from build123d import *

# Parameters (mm, degrees)
F0_R     = 0.6
F1_DEPTH = 1.7
F3_DEPTH = 2
F5_DEPTH = 1
F6_R     = 1.1
F7_DEPTH = 2.701
F8_R     = 2.35
F9_DEPTH = 2


with BuildPart() as f1:
    # F0 (on Top) → F1 (new body)
    with BuildSketch(Plane.XY):
        with BuildLine():
            ThreePointArc((2.2299103121, -2.5), (3.057180036, -1.369726333), (3.35, 0))
            ThreePointArc((3.35, 0), (3.057180036, 1.369726333), (2.2299103121, 2.5))
            ThreePointArc((2.2299103121, 2.5), (-3.35, 0), (2.2299103121, -2.5))
        make_face()
        with BuildLine():
            ThreePointArc((2.2299103121, 2.5), (3.057180036, 1.369726333), (3.35, 0))
            ThreePointArc((3.35, 0), (3.057180036, -1.369726333), (2.2299103121, -2.5))
            Line((2.2299103121, -2.5), (14, -2))
            ThreePointArc((14, -2), (16, 0), (14, 2))
            Line((14, 2), (2.2299103121, 2.5))
        make_face()
        with Locations((4, 0)):
            Circle(F0_R, mode=Mode.SUBTRACT)
        with Locations((6, 0)):
            Circle(F0_R, mode=Mode.SUBTRACT)
        with Locations((8, 0)):
            Circle(F0_R, mode=Mode.SUBTRACT)
        with Locations((10, 0)):
            Circle(F0_R, mode=Mode.SUBTRACT)
        with Locations((12, 0)):
            Circle(F0_R, mode=Mode.SUBTRACT)
        with Locations((14, 0)):
            Circle(F0_R, mode=Mode.SUBTRACT)
    extrude(amount=F1_DEPTH)

    # F2 (on face) → F3 (join)
    with BuildSketch(Plane.XY.offset(1.7)):
        with BuildLine():
            ThreePointArc((2.2299103121, -2.5), (3.35, 0), (2.2299103121, 2.5))
            ThreePointArc((2.2299103121, 2.5), (-3.35, 0), (2.2299103121, -2.5))
        make_face()
    extrude(amount=F3_DEPTH)

    # F4 (on face) → F5 (cut)
    with BuildSketch(Plane(origin=(0, 0, 0), x_dir=(1, 0, 0), z_dir=(0, 0, -1))):
        with BuildLine():
            ThreePointArc((1.5642654428, 1.7537313433), (-2.35, 0), (1.5642654428, -1.7537313433))
            ThreePointArc((1.5642654428, -1.7537313433), (2.35, 0), (1.5642654428, 1.7537313433))
        make_face()
    extrude(amount=-F5_DEPTH, mode=Mode.SUBTRACT)

    # F6 (on face) → F7 (cut, through all)
    with BuildSketch(Plane(origin=(0, 0, 1), x_dir=(1, 0, 0), z_dir=(0, 0, -1))):
        Circle(F6_R)
    extrude(amount=-F7_DEPTH, mode=Mode.SUBTRACT)

    # F8 (on face) → F9 (cut, through all)
    with BuildSketch(Plane.XY.offset(3.7)):
        Circle(F8_R)
    extrude(amount=-F9_DEPTH, mode=Mode.SUBTRACT)


solid = f1.part
Geometry check sheet. Reference: the model listing, model coordinates, mm. A direction names the side the tool comes from. Coordinates: 2 decimals unless noted, no trailing zeros. Order: outer loops, then holes, each group sorted by start corner. A loop starts at its lowest first (then second) coordinate and runs counter-clockwise, first axis right, second up. Notation, with made-up numbers: (88, -25.5) - (93, -25.5) arc R25 cw to (93, 1.5) - close; hole circle Ø9 at (25.25, 52). An arc over 180 degrees is marked (long way). One line per item, written item: value.
(1) Release check for a two-part mould opening along Y. For faces 1 (the face through (8.033, -2.254, 0.838)), 2 (the face through (14.554, -0.23, 0.838)), 3 (the face through (2.2, -1.4, 3.7)) record: +Y half, -Y half, draft (parallel to the pull), parting line (faces both ways), or undercut.
Data:
face 1: -Y half
face 2: undercut
face 3: draft
(2) Depth check by flat-ended pin: pin 1 Ø3 at (x, y) = (0.5, -2.5) entering from -Z; pin 2 Ø0.7 at (x, y) = (14, 0) entering from -Z; pin 3 Ø1.4 at (x, y) = (6, 0) entering from +Z; pin 4 Ø3 at (x, y) = (0, 0) entering from -Z. Enter the tip coordinate at first touch or a pass-through.
Data:
pin 1: stops at z = 0
pin 2: passes through
pin 3: stops at z = 1.7
pin 4: stops at z = 1
(3) Sectioned sample at C-C (y = 1.5). Enter the section's corners in (x, z).
Data:
outline: (-3, 0) - (-1.81, 0) - (-1.81, 1) - (1.81, 1) - (1.81, 0) - (15.32, 0) - (15.32, 1.7) - (3, 1.7) - (3, 3.7) - (1.81, 3.7) - (1.81, 1.7) - (-1.81, 1.7) - (-1.81, 3.7) - (-3, 3.7) - close
(4) Thickness scan on probe 1 along Y at (x, z) = (0, 0.5); probe 2 along Z at (x, y) = (6.5, -1); probe 3 along Y at (x, z) = (4, 0.5). Record the ranges inside material, lowest first. Write a range as from..to.
Data:
probe 1: y = -3.35..-2.35, 2.35..3.35
probe 2: z = 0..1.7
probe 3: y = -2.42..-0.6, 0.6..2.42
(5) Access from +Z, -Z, +X, -X, +Y, -Y to the whole of each face (thin tool, end or side, straight path). Record for faces 4 (the face through (1, -1, 1)), 5 (the face through (16, 0, 1)), 6 (the face through (-0.509, -2.294, 2.714)).
Data:
face 4: -Z
face 5: +Z, -Z, +X
face 6: +Z
(6) Sectioned sample at B-B (x = 10). Enter the section's corners in (y, z), and give its area (3 significant figures).
Data:
outline: (-2.17, 0) - (-0.6, 0) - (-0.6, 1.7) - (-2.17, 1.7) - close; (0.6, 0) - (2.17, 0) - (2.17, 1.7) - (0.6, 1.7) - close
area: 5.34 mm^2
(7) Sectioned sample at D-D (x = 0). Enter the section's corners in (y, z), and give its area (3 significant figures).
Data:
outline: (-3.35, 0) - (-2.35, 0) - (-2.35, 1) - (-1.1, 1) - (-1.1, 1.7) - (-2.35, 1.7) - (-2.35, 3.7) - (-3.35, 3.7) - close; (1.1, 1) - (2.35, 1) - (2.35, 0) - (3.35, 0) - (3.35, 3.7) - (2.35, 3.7) - (2.35, 1.7) - (1.1, 1.7) - close
area: 9.15 mm^2
(8) Sectioned sample at A-A (z = 1.5). Enter the section's corners in (x, y), and give its area (3 significant figures).
Data:
outline: (2.23, -2.5) - (14, -2) arc R2 ccw to (14, 2) - (2.23, 2.5) arc R3.35 ccw (long way) to start; hole circle Ø2.2 at (0, 0); hole circle Ø1.2 at (4, 0); hole circle Ø1.2 at (6, 0); hole circle Ø1.2 at (8, 0); hole circle Ø1.2 at (10, 0); hole circle Ø1.2 at (12, 0); hole circle Ø1.2 at (14, 0)
area: 80.0 mm^2
